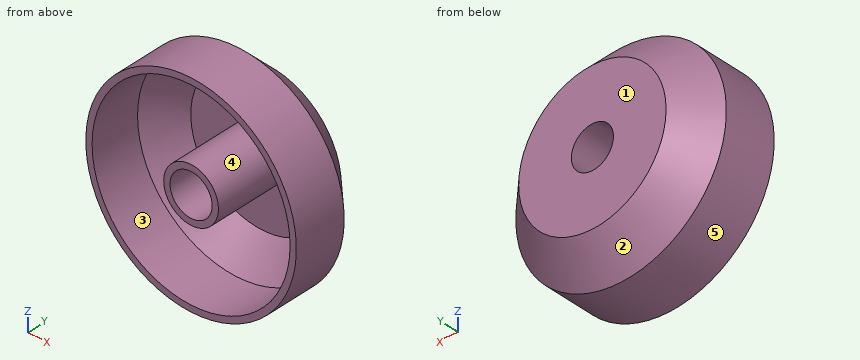
```python
from build123d import *

# Parameters (mm, degrees)
CROQUIS1_R              = 50
CROQUIS1_R_2            = 10
SALIENTE_EXTRUIR1_DEPTH = 40
CHAFL_N1_SIZE           = 15
VACIADO1_T              = -3


with BuildPart() as part:
    # Croquis1 → Saliente-Extruir1 (new body)
    with BuildSketch(Plane(origin=(0, 0, 0), x_dir=(1, 0, 0), z_dir=(0, 1, 0))):
        with Locations(Location((0, 0, 0), (0, 0, 270))):
            Circle(CROQUIS1_R)
        with Locations(Location((0, 0, 0), (0, 0, 270))):
            Circle(CROQUIS1_R_2, mode=Mode.SUBTRACT)
    extrude(amount=SALIENTE_EXTRUIR1_DEPTH)

    # Chaflán1
    chafl_n1_edges = [part.edges().sort_by_distance(p)[0] for p in [
        (0, 40, -50),
    ]]
    chamfer(chafl_n1_edges, length=CHAFL_N1_SIZE)

    # Vaciado1
    vaciado1_openings = [part.faces().sort_by_distance(p)[0] for p in [
        (0, 0, -48.585786438),
    ]]
    offset(amount=VACIADO1_T, openings=vaciado1_openings, kind=Kind.INTERSECTION)


solid = part.part
```
Build history of the part. All positions in model axes, mm. Face numbers are marked on the shaded views. A direction names the side the tool comes from. Round coordinates to 2 decimals unless told otherwise and drop trailing zeros. Write each loop counter-clockwise with the first axis right and the second up, starting at its lowest first coordinate (ties: lowest second). Pieces come first, ordered by that corner, then holes.
1) Drill centre lines: probe 1 along X at (y, z) = (16.5, 0); probe 2 along X at (y, z) = (27.5, 0); probe 3 along Z at (x, y) = (-43, 21). Where is each one in solid material? Low to high.
2) Mould opens along Z. For the marked faces 1, 2 and 3 say: +Z half, -Z half, draft (parallel to the pull), parting line (faces both ways), or undercut.
3) Pin check, flat tips, straight feed: pin 1 (8 mm diameter, centred on x = -33.5, z = 24.5, fed in from -Y); pin 2 (2 mm diameter, centred on y = 25.5, z = -13.5, fed in from -X); pin 3 (1 mm diameter, centred on x = 5.5, z = 34, fed in from -Y). Stop position of each tip, or through.
4) Band-saw the part on A-A, the plane x = 0. List the corners of the cut face in (y, z), and give its area (3 significant figures).
5) Band-saw the part on C-C, the plane y = 18. List the corners of the cut face in (x, z).
6) Band-saw the part on D-D, the plane y = 28.5. List the corners of the cut face in (x, z), and give its area (3 significant figures).
7) 3-axis set-ups, long thin cutter, end or side, ignore diameter. For the marked faces 4 and 5: which of +Z, -Z, +X, -X, +Y, -Y reach the whole face in a straight line?
8) Band-saw the part on B-B, the plane z = 0. List the corners of the cut face in (x, y).
Ans:
1. probe 1: x = -50 to -47, -13 to -10, 10 to 13, 47 to 50
1. probe 2: x = -47.5 to -43.26, -13 to -10, 10 to 13, 43.26 to 47.5
1. probe 3: z = -25.51 to -18.97, 18.97 to 25.51
2. face 1: draft
2. face 2: parting line
2. face 3: undercut
3. pin 1: stops at y = 25.25
3. pin 2: stops at x = -48.38
3. pin 3: stops at y = 35.82
4. outline: (0, -50) - (25, -50) - (40, -35) - (40, -10) - (0, -10) - (0, -13) - (37, -13) - (37, -33.76) - (23.76, -47) - (0, -47) - close; (0, 10) - (40, 10) - (40, 35) - (25, 50) - (0, 50) - (0, 47) - (23.76, 47) - (37, 33.76) - (37, 13) - (0, 13) - close
4. area: 634 mm2
5. outline: circle Ø100 at (0, 0); circle Ø26 at (0, 0); hole circle Ø94 at (0, 0); hole circle Ø20 at (0, 0)
6. outline: circle Ø93 at (0, 0); circle Ø26 at (0, 0); hole circle Ø84.51 at (0, 0); hole circle Ø20 at (0, 0)
6. area: 1,400 mm2
7. face 4: -Y
7. face 5: +Y, -Y
8. outline: (-50, 0) - (-47, 0) - (-47, 23.76) - (-33.76, 37) - (-13, 37) - (-13, 0) - (-10, 0) - (-10, 40) - (-35, 40) - (-50, 25) - close; (10, 0) - (13, 0) - (13, 37) - (33.76, 37) - (47, 23.76) - (47, 0) - (50, 0) - (50, 25) - (35, 40) - (10, 40) - close
